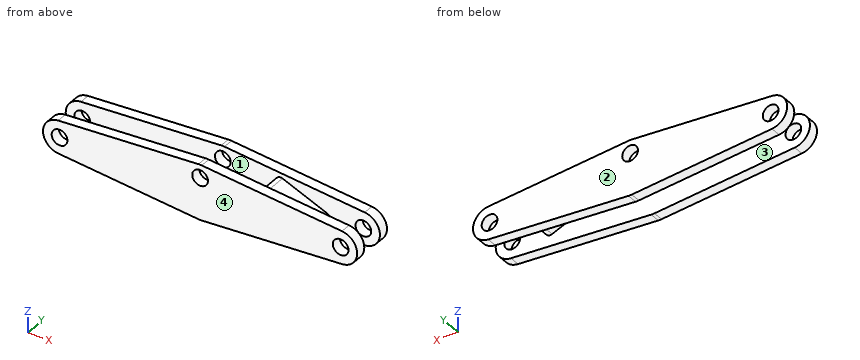
```python
from build123d import *

# Parameters (mm, degrees)
SKETCH1_R                = 4.75
BOSS_EXTRUDE1_DEPTH      = 13.125
SKETCH2_W                = 190
SKETCH2_H                = 13.75
CUT_EXTRUDE1_DEPTH       = 34.711010303
BOSS_EXTRUDE4_DEPTH      = 6.875
BOSS_EXTRUDE4_DEPTH_BACK = 6.875


with BuildPart() as part:
    # Sketch1 → Boss-Extrude1 (new body, symmetric)
    with BuildSketch(Plane(origin=(0, 0, 0), x_dir=(1, 0, 0), z_dir=(0, 1, 0))):
        with BuildLine():
            Line((-0.984987686, 16.672141843), (-85.787990149, 9.968905232))
            ThreePointArc((-85.787990149, 9.968905232), (-95, 0), (-85.787990149, -9.968905232))
            Line((-85.787990149, -9.968905232), (-0.984987686, -16.672141843))
            ThreePointArc((-0.984987686, -16.672141843), (0, -16.711010303), (0.984987686, -16.672141843))
            Line((0.984987686, -16.672141843), (85.787990149, -9.968905232))
            ThreePointArc((85.787990149, -9.968905232), (95, 0), (85.787990149, 9.968905232))
            Line((85.787990149, 9.968905232), (0.984987686, 16.672141843))
            ThreePointArc((0.984987686, 16.672141843), (0, 16.711010303), (-0.984987686, 16.672141843))
        make_face()
        with Locations((-85, 0)):
            Circle(SKETCH1_R, mode=Mode.SUBTRACT)
        with Locations((85, 0)):
            Circle(SKETCH1_R, mode=Mode.SUBTRACT)
        with Locations((0, -8.75)):
            Circle(SKETCH1_R, mode=Mode.SUBTRACT)
    extrude(amount=BOSS_EXTRUDE1_DEPTH, both=True)

    # Sketch2 → Cut-Extrude1 (cut, through all)
    with BuildSketch(Plane.XY.offset(17)):
        Rectangle(SKETCH2_W, SKETCH2_H)
    extrude(amount=-CUT_EXTRUDE1_DEPTH, mode=Mode.SUBTRACT)

    # Sketch3 → Boss-Extrude4 (add, two sides)
    with BuildSketch(Plane(origin=(0, 0, 0), x_dir=(1, 0, 0), z_dir=(0, 1, 0))) as boss_extrude4_sk:
        with BuildLine():
            Line((33.907114097, -5.520713265), (60.914335229, 5.043850462))
            ThreePointArc((60.914335229, 5.043850462), (64.801071594, 3.342885903), (63.100107035, -0.543850462))
            Line((63.100107035, -0.543850462), (36.092885903, -11.108414189))
            ThreePointArc((36.092885903, -11.108414189), (32.206149538, -9.40744963), (33.907114097, -5.520713265))
        make_face()
    extrude(amount=BOSS_EXTRUDE4_DEPTH)
    extrude(boss_extrude4_sk.sketch, amount=-BOSS_EXTRUDE4_DEPTH_BACK)


solid = part.part
```
For this review, take the finished solid that the model builds, in its own axes (mm). Face numbers are marked on the shaded views. Round coordinates to 2 decimals unless told otherwise and drop trailing zeros. Write each loop counter-clockwise with the first axis right and the second up, starting at its lowest first coordinate (ties: lowest second). Pieces come first, ordered by that corner, then holes. Notation, with made-up numbers: M -11,33.5 L 21,33.5 A25 cw 21,65.5 Z; hole C 75,82.25 d11. An arc over 180 degrees is marked long. One line per item, written item: value. Start each with the question number.
(1) We need section A-A (x = 6.5). Give the boundary of the cut face in (y, z) (3 decimals).
(2) Wall thickness on line 1 (Y direction, x = -23.5, z = 13) (3 decimals); line 2 (Z direction, x = 0, y = -10); line 3 (Z direction, x = 85, y = 10): over which ranges is each line inside the solid? List them lowest first.
(3) We need section C-C (z = -2.25). Give the boundary of the cut face in (x, y) (3 decimals), and give its area (3 significant figures).
(4) The part is to be moulded in two halves that separate along Y. For the marked faces 1, 2, 3 and 4, say which applies: released by +Y, released by -Y, zero draft, split by the parting line, or undercut.
(5) We need section D-D (y = 4.25). Give the boundary of the cut face in (x, z).
(6) Insertion check: pin 1 (7.5 mm diameter, centred on x = -85, z = 0, fed in from -Y); pin 2 (5 mm diameter, centred on y = -10.5, z = 11.5, fed in from +X); pin 3 (10 mm diameter, centred on x = -18, y = 3.5, fed in from -Z); pin 4 (1.5 mm diameter, centred on x = -63.5, y = -10.5, fed in from -Z). Each pin has a flat end and moves straight along its axis. Give the tip position at first contact, or say it passes through.
(7) We need section B-B (x = 83.5). Give the boundary of the cut face in (y, z) (3 decimals), and give its area (3 significant figures).
Result:
1. outline: M -13.125,-16.236 L -6.875,-16.236 L -6.875,16.236 L -13.125,16.236 Z; M 6.875,-16.236 L 13.125,-16.236 L 13.125,16.236 L 6.875,16.236 Z
2. line 1: -13.125 to -6.875, 6.875 to 13.125
2. line 2: -16.71 to 4, 13.5 to 16.71
2. line 3: -10.03 to -4.75, 4.75 to 10.03
3. outline: M -94.744,-13.125 L -89.183,-13.125 L -89.183,-6.875 L -94.744,-6.875 Z; M -94.744,6.875 L -89.183,6.875 L -89.183,13.125 L -94.744,13.125 Z; M -80.817,-13.125 L 80.817,-13.125 L 80.817,-6.875 L 65.007,-6.875 L 65.007,6.875 L 80.817,6.875 L 80.817,13.125 L -80.817,13.125 L -80.817,6.875 L 53.772,6.875 L 53.772,-6.875 L -80.817,-6.875 Z; M 89.183,-13.125 L 94.744,-13.125 L 94.744,-6.875 L 89.183,-6.875 Z; M 89.183,6.875 L 94.744,6.875 L 94.744,13.125 L 89.183,13.125 Z
3. area: 2,310 mm²
4. face 1: undercut
4. face 2: released by +Y
4. face 3: undercut
4. face 4: released by -Y
5. outline: M 33.91,5.52 L 60.91,-5.04 A3 ccw 63.1,0.54 L 36.09,11.11 A3 ccw Z
6. pin 1: through
6. pin 2: x = 89.36
6. pin 3: z = -15.62
6. pin 4: z = -11.79
7. outline: M -13.125,-10.15 L -6.875,-10.15 L -6.875,-4.507 L -13.125,-4.507 Z; M -13.125,4.507 L -6.875,4.507 L -6.875,10.15 L -13.125,10.15 Z; M 6.875,-10.15 L 13.125,-10.15 L 13.125,-4.507 L 6.875,-4.507 Z; M 6.875,4.507 L 13.125,4.507 L 13.125,10.15 L 6.875,10.15 Z
7. area: 141 mm²
